Design review of the part built by this model. Coordinates are the model's own, in mm. A direction names the side the tool comes from. Coordinates: 2 decimals unless noted, no trailing zeros. Loops run counter-clockwise (first coordinate to the right, second up) from the corner with the lowest first, then second, coordinate; pieces in that order, holes last. Notation, with made-up numbers: (51, 5.5) -> (106, 5.5) arc R30 ccw to (106, 30.5) -> close; hole circle Ø8 at (46.25, 29). An arc over 180 degrees is marked (long way). One line per item, written item: value. Start each with the question number.
1. Add section A-A on y = 12.7. Write out the cut boundary in (x, z), plus the area to 3 significant figures.
2. Draft analysis for pull direction Y (two halves, no side actions). For faces 4 (the flat face through (-11, -1.27, -11)), 5 (the flat face through (-1, 9.258, -15)), 6 (the flat face through (-14.58, 26.03, -14.95)), state which applies: pulls with the +Y half, pulls with the -Y half, needs draft (parallel to the pull), parting line crosses it, or undercut.
3. Insertion check: pin 1 (5 mm diameter, centred on x = -23, y = 5.5, fed in from +Z); pin 2 (12.5 mm diameter, centred on y = 17, z = -12, fed in from -X); pin 3 (5 mm diameter, centred on y = 13.5, z = -17, fed in from -X); pin 4 (1 mm diameter, centred on x = -11.5, y = 17.5, fed in from -Z). Each pin has a flat end and moves straight along its axis. Give the tip position at first contact, or say it passes through.
4. For probe 1 along Y at (x, z) = (-14.25, -12.75); probe 2 along Z at (x, y) = (-8.75, 11), list the stretches that pass through material, from the lowest coordinate up.
5. Machinability: for faces 1 (the flat face through (-1, 16.142, -15)), 2 (the flat face through (-9, 0, -9)), 3 (the flat face through (-14, 16, 0)), which of the approach directions +Z, -Z, +X, -X, +Y, -Y give a long, thin tool a straight path to every point of the face, cutting with its end or side? Answer none if there is none.
6. Add section B-B on z = -19. Write out the cut boundary in (x, y), plus the area to 3 significant figures.
7. Add section D-D on x = -5. Write out the cut boundary in (y, z), plus the area to 3 significant figures.
8. Add section C-C on y = 2. Write out the cut boundary in (x, z), plus the area to 3 significant figures.
```python
from build123d import *

# Parameters (mm, degrees)
BOSS_EXTRUDE1_DEPTH = 25.4
BOSS_EXTRUDE2_DEPTH = 1.27
BOSS_EXTRUDE3_DEPTH = 1.27
CUT_EXTRUDE1_DEPTH  = 47.758814744
SKETCH5_R           = 3.175
CUT_EXTRUDE2_DEPTH  = 47.758814744


with BuildPart() as part:
    # Sketch1 → Boss-Extrude1 (new body)
    with BuildSketch(Plane(origin=(0, 0, 0), x_dir=(1, 0, 0), z_dir=(0, 1, 0))):
        Polygon((-27.94, 1.5875), (-1.5875, 1.5875), (-1.5875, 27.94), (0, 27.94), (0, 0), (-27.94, 0), align=None)
    extrude(amount=BOSS_EXTRUDE1_DEPTH)

    # Sketch2 → Boss-Extrude2 (add)
    with BuildSketch(Plane(origin=(0, 25.4, 0), x_dir=(1, 0, 0), z_dir=(0, 1, 0))):
        Polygon((-1.5875, 27.94), (-27.94, 1.5875), (-27.94, 0), (0, 0), (0, 27.94), align=None)
    extrude(amount=BOSS_EXTRUDE2_DEPTH)

    # Sketch3 → Boss-Extrude3 (add)
    with BuildSketch(Plane.XZ):
        Polygon((-27.94, -1.5875), (-1.5875, -27.94), (0, -27.94), (0, 0), (-27.94, 0), align=None)
    extrude(amount=BOSS_EXTRUDE3_DEPTH)

    # Sketch4 → Cut-Extrude1 (cut, through all)
    with BuildSketch(Plane.ZY.offset(1.5875)):
        with BuildLine():
            Line((-20.32, 9.2583), (-9.2075, 9.2583))
            ThreePointArc((-9.2075, 9.2583), (-5.7658, 12.7), (-9.2075, 16.1417))
            Line((-9.2075, 16.1417), (-20.32, 16.1417))
            ThreePointArc((-20.32, 16.1417), (-23.7617, 12.7), (-20.32, 9.2583))
        make_face()
    extrude(amount=-CUT_EXTRUDE1_DEPTH, mode=Mode.SUBTRACT)

    # Sketch5 → Cut-Extrude2 (cut, through all)
    with BuildSketch(Plane(origin=(0, 0, -1.5875), x_dir=(-1, 0, 0), z_dir=(0, 0, -1))):
        with Locations((14.76375, 12.7)):
            Circle(SKETCH5_R)
    extrude(amount=-CUT_EXTRUDE2_DEPTH, mode=Mode.SUBTRACT)


solid = part.part
```
Worked answers:
1. outline: (-27.94, -1.59) -> (-17.94, -1.59) -> (-17.94, 0) -> (-27.94, 0) -> close; (-11.59, -1.59) -> (-1.59, -1.59) -> (-1.59, -5.77) -> (0, -5.77) -> (0, 0) -> (-11.59, 0) -> close; (-1.59, -27.94) -> (0, -27.94) -> (0, -23.76) -> (-1.59, -23.76) -> close
1. area: 47.5 mm²
2. face 4: pulls with the -Y half
2. face 5: undercut
2. face 6: needs draft
3. pin 1: stops at z = 0
3. pin 2: stops at x = -1.59
3. pin 3: passes through
3. pin 4: stops at z = -1.59
4. probe 1: y = -1.27 to 0, 25.4 to 26.67
4. probe 2: z = -1.59 to 0
5. face 1: +X, -X
5. face 2: -Z, -X
5. face 3: +Z, +X, -X, +Y, -Y
6. outline: (-10.53, -1.27) -> (0, -1.27) -> (0, 9.26) -> (-1.59, 9.26) -> (-1.59, 0) -> (-10.53, 0) -> close; (-10.53, 25.4) -> (-1.59, 25.4) -> (-1.59, 16.14) -> (0, 16.14) -> (0, 26.67) -> (-10.53, 26.67) -> close
6. area: 56.1 mm²
7. outline: (-1.27, -24.53) -> (0, -24.53) -> (0, -1.59) -> (25.4, -1.59) -> (25.4, -24.53) -> (26.67, -24.53) -> (26.67, 0) -> (-1.27, 0) -> close
7. area: 103 mm²
8. outline: (-27.94, -1.59) -> (-1.59, -1.59) -> (-1.59, -27.94) -> (0, -27.94) -> (0, 0) -> (-27.94, 0) -> close
8. area: 86.2 mm²
